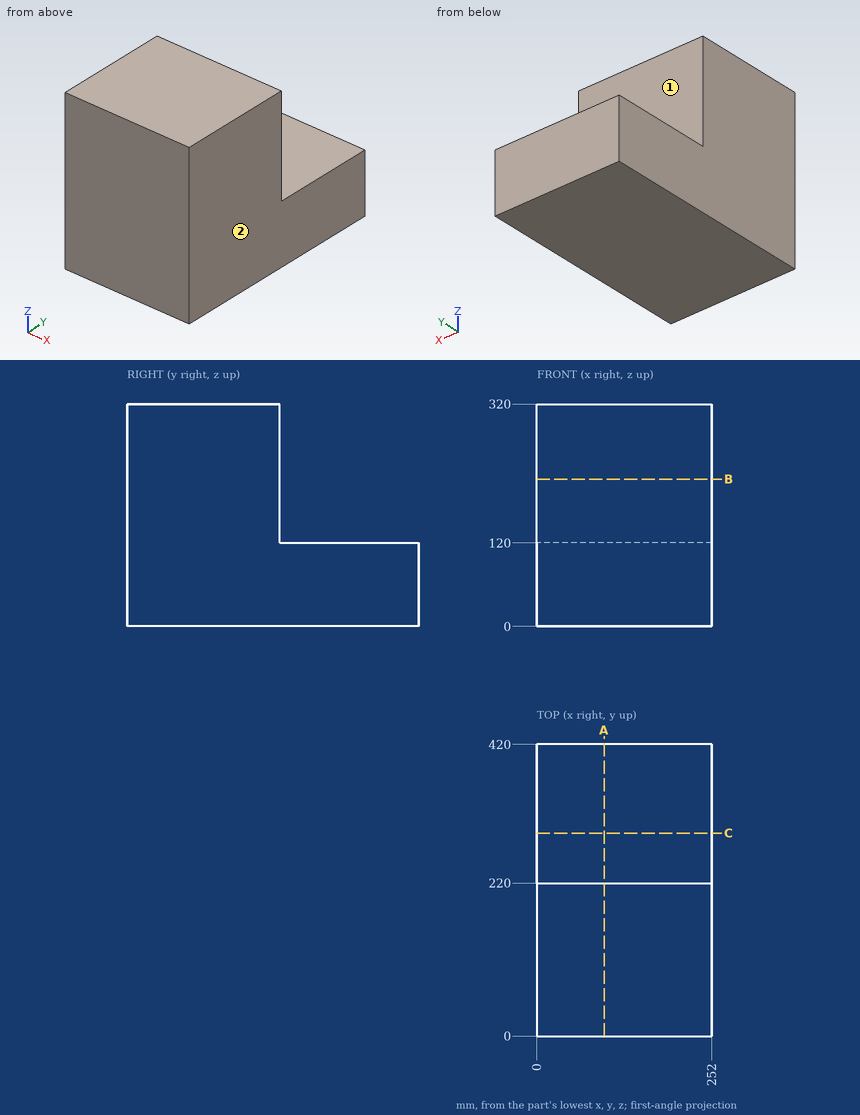
Part print with two shaded views. Sizes in mm from the minimum x, y, z corner. A direction names the side the tool comes from. Coordinates: 2 decimals unless noted, no trailing zeros. Order: outer loops, then holes, each group sorted by start corner. A loop starts at its lowest first (then second) coordinate and runs counter-clockwise, first axis right, second up. Notation, with made-up numbers: M 85.5,82 L 125.5,82 A25 cw 125.5,114 Z; hole C -36,23 d11. An arc over 180 degrees is marked long. One line per question, with ' | ' between items. Start each with the question number.
1. Wall check: line 1 along Y through (x, z) = (121.5, 193.5); line 2 along Z through (x, y) = (47, 298.5). Give the ranges that are in metal, low to high. Write a range as [from, to].
2. Tool access for the marked faces 1 and 2: list every direction of +Z, -Z, +X, -X, +Y, -Y with a clear straight run to the whole face (end or side of a thin tool).
3. Cut at C-C (y = 292). Write the cut outline in (x, z).
4. Cut at B-B (z = 212). Write the cut outline in (x, y).
5. Cut at A-A (x = 97). Write the cut outline in (y, z).
The answers:
1) line 1: y = [0, 220] | line 2: z = [0, 120]
2) face 1: +Z, +X, -X, +Y | face 2: +Z, -Z, +X, +Y, -Y
3) outline: M 0,0 L 252,0 L 252,120 L 0,120 Z
4) outline: M 0,0 L 252,0 L 252,220 L 0,220 Z
5) outline: M 0,0 L 420,0 L 420,120 L 220,120 L 220,320 L 0,320 Z
